```python
from build123d import *

# Parameters (mm, degrees)
SKETCH1_R           = 85
SKETCH1_R_2         = 83
EXTRUDE_THIN1_DEPTH = 450
SKETCH2_R           = 7.5
CUT_EXTRUDE1_DEPTH  = 100
CIRPATTERN1_COUNT   = 2
CIRPATTERN1_ANGLE   = 90


with BuildPart() as part:
    # Sketch1 → Extrude-Thin1 (new body)
    with BuildSketch(Plane(origin=(0, 0, 0), x_dir=(1, 0, 0), z_dir=(0, 1, 0))):
        Circle(SKETCH1_R)
        Circle(SKETCH1_R_2, mode=Mode.SUBTRACT)
    extrude(amount=EXTRUDE_THIN1_DEPTH)

    # Sketch2 → Cut-Extrude1 (cut, symmetric)
    with BuildSketch(Plane.XY):
        with Locations((0, 32.7)):
            Circle(SKETCH2_R)
    cut_extrude1 = extrude(amount=CUT_EXTRUDE1_DEPTH, both=True, mode=Mode.SUBTRACT)

    # CirPattern1: Cut-Extrude1 ×2 about axis
    cirpattern1_axis = Axis((0, 450, 0), (0, -1, 0))
    for i in range(1, CIRPATTERN1_COUNT):
        add(cut_extrude1.rotate(cirpattern1_axis, i * CIRPATTERN1_ANGLE / (CIRPATTERN1_COUNT - 1)), mode=Mode.SUBTRACT)


solid = part.part
```
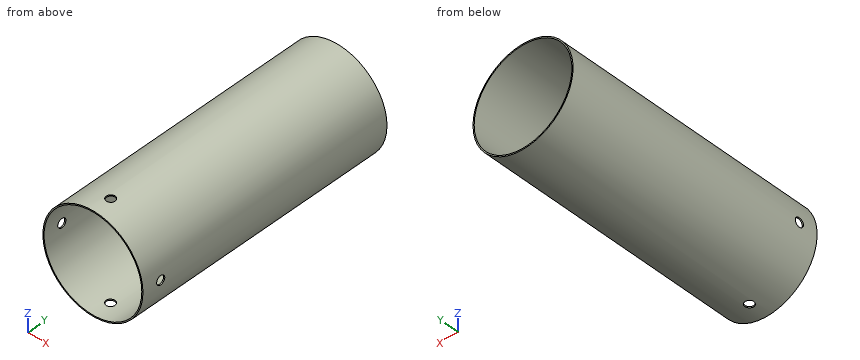
Read the model definition and answer for the solid it produces. Units are mm, in the model's axes. Coordinates: 2 decimals unless noted, no trailing zeros. Loops run counter-clockwise (first coordinate to the right, second up) from the corner with the lowest first, then second, coordinate; pieces in that order, holes last. Notation, with made-up numbers: (-1, 60.5) -> (33, 60.5) arc R20 ccw to (33, 97.5) -> close; hole circle Ø4 at (76, 53). An arc over 180 degrees is marked (long way). Return JSON: item names as keys, results as strings.
Item 1: Find section A-A (z = 0). Determine the outline of the cut face in (x, y), plus the area to 3 significant figures.
Answers:
{"outline": "(-85, 0) -> (-83, 0) -> (-83, 25.2) -> (-85, 25.2) -> close; (-85, 40.2) -> (-83, 40.2) -> (-83, 450) -> (-85, 450) -> close; (83, 0) -> (85, 0) -> (85, 25.2) -> (83, 25.2) -> close; (83, 40.2) -> (85, 40.2) -> (85, 450) -> (83, 450) -> close", "area": "1,740 mm2"}
Item 2: Find the intervals of material crossed by probe 1 along X at (y, z) = (54, -1); probe 2 along Y at (x, z) = (84.3, 0); probe 3 along X at (y, z) = (181, -67.5), in increasing order.
Answers:
{"probe 1": "x = -84.99 to -82.99, 82.99 to 84.99", "probe 2": "y = 0 to 25.2, 40.2 to 450", "probe 3": "x = -51.66 to -48.3, 48.3 to 51.66"}
Item 3: Find section B-B (x = 0). Determine the outline of the cut face in (y, z).
Answers:
{"outline": "(0, -85) -> (25.2, -85) -> (25.2, -83) -> (0, -83) -> close; (0, 83) -> (25.2, 83) -> (25.2, 85) -> (0, 85) -> close; (40.2, -85) -> (450, -85) -> (450, -83) -> (40.2, -83) -> close; (40.2, 83) -> (450, 83) -> (450, 85) -> (40.2, 85) -> close"}
Item 4: Find section C-C (x = -62). Determine the outline of the cut face in (y, z), plus the area to 3 significant figures.
Answers:
{"outline": "(0, -58.15) -> (450, -58.15) -> (450, -55.18) -> (0, -55.18) -> close; (0, 55.18) -> (450, 55.18) -> (450, 58.15) -> (0, 58.15) -> close", "area": "2,670 mm2"}
Item 5: Find section D-D (z = -41). Determine the outline of the cut face in (x, y), plus the area to 3 significant figures.
Answers:
{"outline": "(-74.46, 0) -> (-72.17, 0) -> (-72.17, 450) -> (-74.46, 450) -> close; (72.17, 0) -> (74.46, 0) -> (74.46, 450) -> (72.17, 450) -> close", "area": "2,060 mm2"}
Item 6: Flat-ended cylindrical pins translate along their axes: P1, Ø12, axis at x = 0, y = 32.7, coming from the +Z side; P2, Ø1.5, axis at y = 263.5, z = -13, coming from the -X side; P3, Ø4, axis at x = 8, y = 131.5, coming from the -Z side; P4, Ø24, axis at y = 32.7, z = 0, coming from the -X side. Find the tip coordinate at first contact, or state that the pin passes through.
Answers:
{"P1": "passes through", "P2": "stops at x = -84.11", "P3": "stops at z = -84.79", "P4": "stops at x = -85"}
